Here's how the part is built. I have some questions about the finished solid (model axes, mm). Coordinates: 2 decimals unless noted, no trailing zeros. Write each loop counter-clockwise with the first axis right and the second up, starting at its lowest first coordinate (ties: lowest second). Pieces come first, ordered by that corner, then holes. Notation, with made-up numbers: M 16,3.25 L 31,3.25 A22 cw 31,35.25 Z; hole C 42.25,-3.75 d8. An arc over 180 degrees is marked long. Use a Markdown table: item, result.
```python
from build123d import *

# Parameters (mm, degrees)
SKETCH_1_R      = 3
SKETCH_1_R_2    = 1.1
EXTRUDE_1_DEPTH = 2.5
CHAMFER_1_SIZE  = 0.1


with BuildPart() as part:
    # ｽｹｯﾁ1 → ﾎﾞｽ - 押し出し1 (new, symmetric)
    with BuildSketch(Plane(origin=(0, 0, 0), x_dir=(1, 0, 0), z_dir=(0, 1, 0))):
        with Locations(Location((0, 0, 0), (0, 0, 270))):
            Circle(SKETCH_1_R)
        with Locations(Location((0, 0, 0), (0, 0, 270))):
            Circle(SKETCH_1_R_2, mode=Mode.SUBTRACT)
    extrude(amount=EXTRUDE_1_DEPTH, both=True)

    # 面取り1
    chamfer_1_edges = [part.edges().sort_by_distance(p)[0] for p in [
        (0, -2.5, -3),
        (0, 2.5, -3),
        (0, -2.5, -1.1),
        (0, 2.5, -1.1),
    ]]
    chamfer(chamfer_1_edges, length=CHAMFER_1_SIZE)


solid = part.part
```
1. Suppose I cut it at C-C on y = 1.65. Write out the boundary of the cut face in (x, z).
Answers follow:
| item | result |
|---|---|
| outline | C 0,0 d6; hole C 0,0 d2.2 |
2. Suppose I cut it at B-B on z = 0. Write out the boundary of the cut face in (x, y).
Answers follow:
| item | result |
|---|---|
| outline | M -3,-2.4 L -2.9,-2.5 L -1.2,-2.5 L -1.1,-2.4 L -1.1,2.4 L -1.2,2.5 L -2.9,2.5 L -3,2.4 Z; M 1.1,-2.4 L 1.2,-2.5 L 2.9,-2.5 L 3,-2.4 L 3,2.4 L 2.9,2.5 L 1.2,2.5 L 1.1,2.4 Z |
3. I need wall thicknesses on probe 1 along X at (y, z) = (-1.3, 0); probe 2 along X at (y, z) = (0.4, -2.4); probe 3 along Z at (x, y) = (0.25, 1.75). Which ranges of each line are inside material? Lowest first, please.
Answers follow:
| item | result |
|---|---|
| probe 1 | x = -3 to -1.1, 1.1 to 3 |
| probe 2 | x = -1.8 to 1.8 |
| probe 3 | z = -2.99 to -1.07, 1.07 to 2.99 |
4. We'd pull the mould along Z, two halves only. Please class faces 1 (the face through (-1, -2.5, 1)), 2 (the face through (0.9, 0.03, 2.86)), 3 (the face through (1.09, -0.03, -0.14)): +Z half, -Z half, draft (parallel to the pull), parting line (faces both ways), or undercut.
Answers follow:
| item | result |
|---|---|
| face 1 | draft |
| face 2 | parting line |
| face 3 | undercut |
5. Suppose I cut it at A-A on x = 0. Write out the boundary of the cut face in (y, z).
Answers follow:
| item | result |
|---|---|
| outline | M -2.5,-2.9 L -2.4,-3 L 2.4,-3 L 2.5,-2.9 L 2.5,-1.2 L 2.4,-1.1 L -2.4,-1.1 L -2.5,-1.2 Z; M -2.5,1.2 L -2.4,1.1 L 2.4,1.1 L 2.5,1.2 L 2.5,2.9 L 2.4,3 L -2.4,3 L -2.5,2.9 Z |
